Can you work these out from the model? Positions are in its coordinate system, mm. A direction names the side the tool comes from. Coordinates: 2 decimals unless noted, no trailing zeros. Order: outer loops, then holes, each group sorted by start corner. A loop starts at its lowest first (then second) coordinate and runs counter-clockwise, first axis right, second up.
```python
from build123d import *

# Parameters (mm, degrees)
SKETCH1_W                = 27.94
SKETCH1_H                = 17.145
BOSS_EXTRUDE1_DEPTH      = 1.016
CUT_EXTRUDE1_DEPTH       = 1.016
BOSS_EXTRUDE2_DEPTH      = 0.762
BOSS_EXTRUDE2_DEPTH_BACK = 3.556
SKETCH3_R                = 0.508
CHAMFER1_SIZE            = 0.127
SKETCH4_W                = 1.840091878
SKETCH4_H                = 0.995012645
SKETCH4_W_2              = 1.93550405
SKETCH4_W_3              = 1.540225054
SKETCH4_H_2              = 1.049533886
SKETCH4_W_4              = 1.526594744
SKETCH4_W_5              = 2.507977079
SKETCH4_H_3              = 1.58793114
SKETCH4_W_6              = 1.022273265
SKETCH4_H_4              = 2.044546532
SKETCH4_W_7              = 0.69514582
SKETCH4_H_5              = 1.090424817
SKETCH4_W_8              = 2.317152736
SKETCH4_H_6              = 6.256312386
SKETCH4_W_9              = 1.172206678
SKETCH4_H_7              = 2.153589013
SKETCH4_W_10             = 3.339426002
SKETCH4_H_8              = 4.034571822
SKETCH4_W_11             = 0.626994269
SKETCH4_H_9              = 0.408909306
SKETCH4_W_12             = 1.731049397
SKETCH4_H_10             = 0.899600474
SKETCH4_W_13             = 0.872339854
SKETCH4_H_11             = 1.185836988
BOSS_EXTRUDE4_DEPTH      = 0.762
BOSS_EXTRUDE5_DEPTH      = 2.54


with BuildPart() as part:
    # Sketch1 → Boss-Extrude1 (new body)
    with BuildSketch(Plane(origin=(0, 0, 0), x_dir=(1, 0, 0), z_dir=(0, 1, 0))):
        with Locations((13.97, 8.5725)):
            Rectangle(SKETCH1_W, SKETCH1_H)
    extrude(amount=BOSS_EXTRUDE1_DEPTH)

    # Sketch2 → Cut-Extrude1 (cut)
    with BuildSketch(Plane(origin=(0, 1.016, 0), x_dir=(1, 0, 0), z_dir=(0, 1, 0))):
        with BuildLine():
            Line((0.635, 3.175), (0, 3.175))
            Line((0, 3.175), (0, 3.302))
            Line((0, 3.302), (0, 13.843))
            Line((0, 13.843), (0.650095852, 13.843))
            ThreePointArc((0.650095852, 13.843), (1.094049376, 13.647878234), (1.27, 13.195983763))
            Line((1.27, 13.195983763), (1.27, 3.792909702))
            ThreePointArc((1.27, 3.792909702), (1.080473289, 3.352442045), (0.635, 3.175))
        make_face()
        with BuildLine():
            Line((27.2415, 2.032), (27.94, 2.032))
            Line((27.94, 2.032), (27.94, 15.113))
            Line((27.94, 15.113), (27.2415, 15.113))
            ThreePointArc((27.2415, 15.113), (26.747585913, 14.908414087), (26.543, 14.4145))
            Line((26.543, 14.4145), (26.543, 2.693369934))
            ThreePointArc((26.543, 2.693369934), (26.755275802, 2.21802088), (27.2415, 2.032))
        make_face()
    extrude(amount=-CUT_EXTRUDE1_DEPTH, mode=Mode.SUBTRACT)

    # Sketch3 → Boss-Extrude2 (add, two sides: drawn at the far end of the back side and taken through both)
    with BuildSketch(Plane(origin=(0, 1.016, 0), x_dir=(1, 0, 0), z_dir=(0, 1, 0)).offset(-BOSS_EXTRUDE2_DEPTH_BACK)):
        with Locations(Location((24.384, 15.621, 0), (0, 0, 90))):
            Circle(SKETCH3_R)
        with Locations(Location((24.384, 12.446, 0), (0, 0, 90))):
            Circle(SKETCH3_R)
        with Locations(Location((24.384, 1.905, 0), (0, 0, 90))):
            Circle(SKETCH3_R)
        with Locations(Location((24.384, 5.08, 0), (0, 0, 90))):
            Circle(SKETCH3_R)
        with Locations(Location((1.524, 15.621, 0), (0, 0, 90))):
            Circle(SKETCH3_R)
        with Locations(Location((1.524, 1.905, 0), (0, 0, 90))):
            Circle(SKETCH3_R)
    extrude(amount=BOSS_EXTRUDE2_DEPTH + BOSS_EXTRUDE2_DEPTH_BACK)

    # Chamfer1
    chamfer1_edges = [part.edges().sort_by_distance(p)[0] for p in [
        (1.524, 1.016, -15.113),
        (1.524, 0, -15.113),
        (1.524, -2.54, -15.113),
        (1.524, 1.778, -15.113),
        (1.524, 1.016, -1.397),
        (1.524, 0, -1.397),
        (1.524, -2.54, -1.397),
        (1.524, 1.778, -1.397),
        (24.384, 1.016, -4.572),
        (24.384, 0, -4.572),
        (24.384, -2.54, -4.572),
        (24.384, 1.778, -4.572),
        (24.384, 1.016, -11.938),
        (24.384, 0, -11.938),
        (24.384, -2.54, -11.938),
        (24.384, 1.778, -11.938),
        (24.384, 1.016, -1.397),
        (24.384, 0, -1.397),
        (24.384, -2.54, -1.397),
        (24.384, 1.778, -1.397),
        (24.384, 1.016, -15.113),
        (24.384, 0, -15.113),
        (24.384, -2.54, -15.113),
        (24.384, 1.778, -15.113),
    ]]
    chamfer(chamfer1_edges, length=CHAMFER1_SIZE)

    # Sketch4 → Boss-Extrude4 (add)
    with BuildSketch(Plane(origin=(0, 1.016, 0), x_dir=(1, 0, 0), z_dir=(0, 1, 0))):
        with Locations((5.110298363, 15.32631871)):
            Rectangle(SKETCH4_W, SKETCH4_H)
        with Locations((8.156672695, 15.32631871)):
            Rectangle(SKETCH4_W_2, SKETCH4_H)
        with Locations((5.110298363, 13.799723966)):
            Rectangle(SKETCH4_W_3, SKETCH4_H_2)
        with Locations((8.156672695, 13.799723966)):
            Rectangle(SKETCH4_W_4, SKETCH4_H_2)
        with Locations((21.241770498, 13.005758396)):
            Rectangle(SKETCH4_W_5, SKETCH4_H_3)
        with Locations((18.795129815, 14.40627277)):
            Rectangle(SKETCH4_W_6, SKETCH4_H_4)
        with Locations((18.631566092, 11.666580418)):
            Rectangle(SKETCH4_W_7, SKETCH4_H_5)
        with Locations((21.337182669, 6.425726142)):
            Rectangle(SKETCH4_W_8, SKETCH4_H_6)
        with Locations((18.720163108, 6.268977575)):
            Rectangle(SKETCH4_W_9, SKETCH4_H_7)
        with Locations((7.032172103, 9.104082098)):
            Rectangle(SKETCH4_W_10, SKETCH4_H_8)
        with Locations((4.939919486, 4.606079729)):
            Rectangle(SKETCH4_W_11, SKETCH4_H_9)
        with Locations((8.163487851, 4.360734145)):
            Rectangle(SKETCH4_W_12, SKETCH4_H_10)
        with Locations((16.484792234, 11.618874332)):
            Rectangle(SKETCH4_W_13, SKETCH4_H_11)
    extrude(amount=BOSS_EXTRUDE4_DEPTH)

    # Sketch5 → Boss-Extrude5 (add)
    with BuildSketch(Plane(origin=(0, 1.016, 0), x_dir=(1, 0, 0), z_dir=(0, 1, 0))):
        Polygon((4.445, 12.319), (0, 12.319), (-0.635, 12.319), (-0.635, 4.699), (4.445, 4.699), align=None)
    extrude(amount=BOSS_EXTRUDE5_DEPTH)


solid = part.part
```
1. Thinking about a two-plate mould opening in X: for faces 6 (the flat face through (2, 2, -12.319)), 7 (the flat face through (0, 0.5, -15.5)), 8 (the flat face through (14, 1.016, -9)), which applies, pulls with the +X half, pulls with the -X half, needs draft (parallel to the pull), parting line crosses it, or undercut?
Completed:
face 6: needs draft
face 7: pulls with the -X half
face 8: undercut
2. I'm going to push flat-ended pins straight in: pin 1 (0.8 mm diameter, centred on x = 16.5, y = 1.5, fed in from -Z); pin 2 (1.5 mm diameter, centred on x = 10, z = -3.5, fed in from -Y); pin 3 (1.2 mm diameter, centred on x = 8, z = -14, fed in from +Y). Where does each tip first touch, or does it pass through?
Completed:
pin 1: stops at z = -12.21
pin 2: stops at y = 0
pin 3: stops at y = 1.78
3. On a 3-axis mill with a long thin cutter (end or side, diameter ignored), from which of +Z, -Z, +X, -X, +Y, -Y can I reach the whole of each face in a straight line? I mean faces 1 (the flat face through (2, 3.556, -9)), 2 (the flat face through (19, 1.778, -6)), 3 (the cylindrical face through (24.041, 1.393, -4.706)), 4 (the flat face through (13.8, 0.5, 0)), 5 (the cylindrical face through (23.88, -1.29, -12.38)). Say none if no direction works.
Completed:
face 1: +Z, -Z, +X, -X, +Y
face 2: +Z, -Z, +X, +Y
face 3: +Y
face 4: +Z, +X, -X, +Y, -Y
face 5: -Y
4. Please list where these lines run through material, in increasing order: probe 1 along X at (y, z) = (1.5, -11.5) (3 decimals); probe 2 along Z at (x, y) = (0.5, 0.75) (3 decimals); probe 3 along X at (y, z) = (0.5, -6.5).
Completed:
probe 1: x = -0.635 to 4.445, 16.049 to 16.921, 18.284 to 18.979
probe 2: z = -17.145 to -13.843, -3.175 to 0
probe 3: x = 1.27 to 26.54
5. Imagine slicing it at B-B on x = 9.75. Please give me the cut outline in (y, z) (3 decimals), then the cut area to 3 significant figures.
Completed:
outline: (0, -17.145) - (1.016, -17.145) - (1.016, 0) - (0, 0) - close
area: 17.4 mm2
6. Imagine slicing it at A-A on y = -1.25. Please give me the cut outline in (x, z) (3 decimals).
Completed:
outline: circle Ø1.016 at (1.524, -15.621); circle Ø1.016 at (1.524, -1.905); circle Ø1.016 at (24.384, -15.621); circle Ø1.016 at (24.384, -12.446); circle Ø1.016 at (24.384, -5.08); circle Ø1.016 at (24.384, -1.905)
7. Imagine slicing it at C-C on y = 2.5. Please give me the cut outline in (x, z) (3 decimals), then the cut area to 3 significant figures.
Completed:
outline: (-0.635, -12.319) - (4.445, -12.319) - (4.445, -4.699) - (-0.635, -4.699) - close
area: 38.7 mm2
